Autodesk Fusion 360 part; units mm, degrees
sketch "Sketch1" plane through (0, 0, 0) normal (0, 0, 1) x (1, 0, 0)
  circle A0 centre (0, 0) radius 8
  dimension "d1" = 16
extrude "Extrude1" add sketch "Sketch1" along normal blind 17
sketch "Sketch2" plane through (0, 0, 17) normal (0, 0, 1) x (-1, 0, 0)
  circle A0 centre (0, 0) radius 8
  circle A1 centre (0, 0) radius 10
  dimension "d4" = 20
extrude "Extrude2" add sketch "Sketch2" along normal blind 20 contours A0 | A1
sketch "Sketch3" plane through (0, 0, 0) normal (0, 0, -1) x (1, 0, 0)
  circle A0 centre (0, 0) radius 8
  circle A1 centre (0, 0) radius 5.1
  dimension "d7" = 10.2
extrude "Extrude3" cut sketch "Sketch3" against normal blind 3 contours A1
sketch "Sketch4" plane through (0, 0, 3) normal (0, 0, -1) x (1, 0, 0)
  circle A0 centre (0, 0) radius 5.1
  circle A1 centre (0, 0) radius 2
extrude "Extrude4" cut sketch "Sketch4" against normal up to surface (34 mm away) contours A1
Geometry check sheet. Reference: the model listing, model coordinates, mm. A direction names the side the tool comes from. Round coordinates to 2 decimals unless told otherwise and drop trailing zeros. Write each loop counter-clockwise with the first axis right and the second up, starting at its lowest first coordinate (ties: lowest second). Pieces come first, ordered by that corner, then holes.
Item 1: Material ranges on line 1 along Y through (x, z) = (0, 16.5); line 2 along Z through (x, y) = (3.5, 7.5); line 3 along X through (y, z) = (0, 18), recorded low to high.
Determined:
line 1: y = -8 to -2, 2 to 8
line 2: z = 17 to 37
line 3: x = -10 to -2, 2 to 10
Item 2: Section check A-A (y = 0). Record the boundary of the cut face in (x, z).
Determined:
outline: (-10, 17) - (-8, 17) - (-8, 0) - (-5.1, 0) - (-5.1, 3) - (-2, 3) - (-2, 37) - (-10, 37) - close; (2, 3) - (5.1, 3) - (5.1, 0) - (8, 0) - (8, 17) - (10, 17) - (10, 37) - (2, 37) - close
Item 3: Access from +Z, -Z, +X, -X, +Y, -Y to the whole of each face (thin tool, end or side, straight path). Record for faces 1 (the face through (2.4, 4.5, 1.5)), 2 (the face through (2.17, -9.76, 26.86)).
Determined:
face 1: -Z
face 2: +Z, -Z
Item 4: Section check C-C (z = 30.5). Record the boundary of the cut face in (x, y).
Determined:
outline: circle Ø20 at (0, 0); hole circle Ø4 at (0, 0)
Item 5: Go/stop test with flat-tipped pins: pin 1 Ø3 at (x, y) = (-1, 7) entering from -Z; pin 2 Ø1 at (x, z) = (-0.5, 15) entering from +Y; pin 3 Ø5 at (y, z) = (5, 8.5) entering from -X; pin 4 Ø3 at (x, z) = (-2, 17) entering from +Y. Record where each tip stops, or that it passes through.
Determined:
pin 1: stops at z = 0
pin 2: stops at y = 8
pin 3: stops at x = -7.6
pin 4: stops at y = 9.99
Item 6: Section check D-D (y = -3). Record the boundary of the cut face in (x, z).
Determined:
outline: (-9.54, 17) - (-7.42, 17) - (-7.42, 0) - (-4.12, 0) - (-4.12, 3) - (4.12, 3) - (4.12, 0) - (7.42, 0) - (7.42, 17) - (9.54, 17) - (9.54, 37) - (-9.54, 37) - close
Item 7: Mould release check, pull along X, two halves, no side actions. Record for faces 3 (the face through (-1.73, 7.81, 8.38)), 4 (the face through (0, 2, 20)), 5 (the face through (0.1, -2.4, 37)): +X half, -X half, draft (parallel to the pull), parting line (faces both ways), or undercut.
Determined:
face 3: parting line
face 4: undercut
face 5: draft
